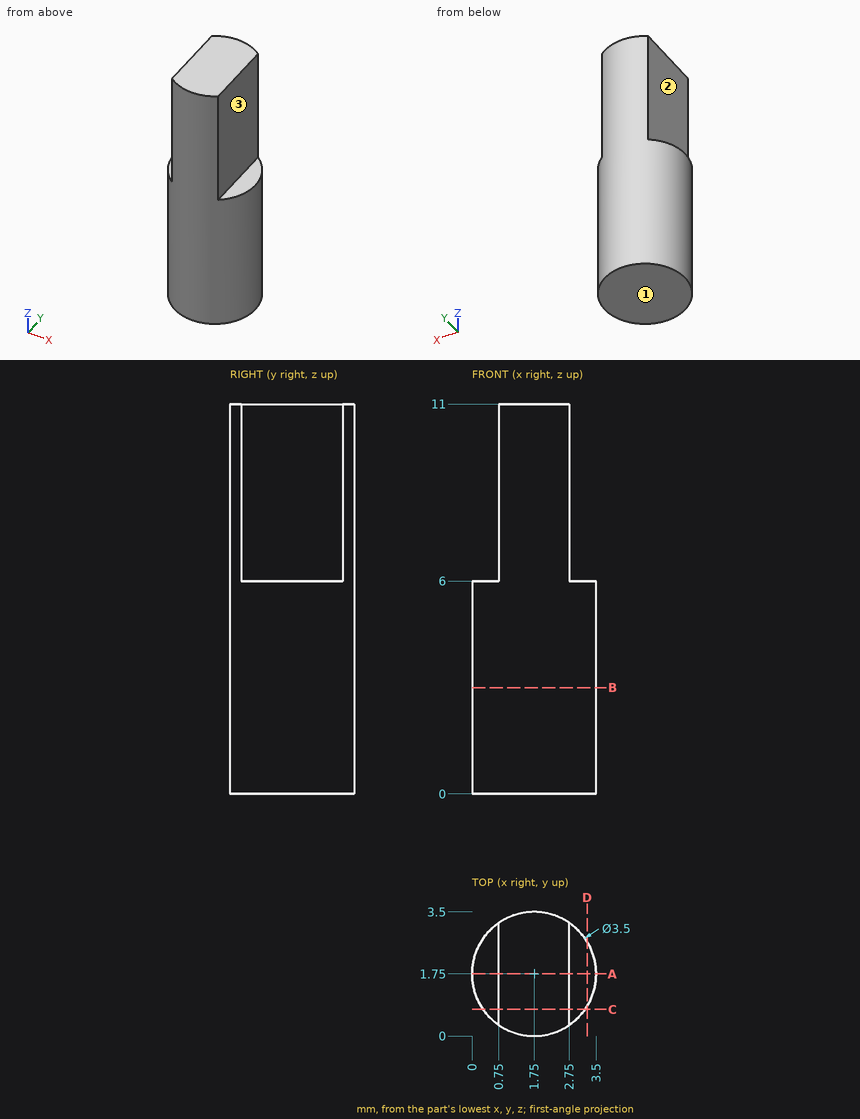
Input: dimensioned drawing with shaded views. Units: mm. Origin: part minimum x, y, z. A direction names the side the tool comes from. Give positions to 0.01 mm unless a question says otherwise; leave off trailing zeros. Loops run counter-clockwise (first coordinate to the right, second up) from the corner with the lowest first, then second, coordinate; pieces in that order, holes last. Notation, with made-up numbers: M 34,31 L 93,31 A19 cw 93,36 Z; hole C 2.25,0.5 d1. An arc over 180 degrees is marked long. Put each result on its own line as item: value. Start each with the question number.
1) Cut plane C-C (y = 0.75). Output: boundary loops of the cut face in (x, z), then the cut area to 3 significant figures.
2) Cut plane D-D (x = 3.25). Output: boundary loops of the cut face in (y, z), then the cut area to 3 significant figures.
3) Ray query, line 1 along X through (y, z) = (0.35, 10.25); line 2 along Z through (x, y) = (3.15, 1.2); line 3 along Y through (x, z) = (1.65, 6.5). Return the intervals inside material, ascending.
4) Contact query for a flat-ended pin moving along its axis: pin 1 (2 mm diameter, centred on y = 0.5, z = 9.5, fed in from +X). Output: stop coordinate, or through.
5) Access query for the marked faces 1, 2 and 3. Directions: +Z, -Z, +X, -X, +Y, -Y. A direction counts if a zero-diameter tool reaches every point of the face in a straight line with its end or side. Return the directions, or none.
6) Cut plane B-B (z = 3). Output: boundary loops of the cut face in (x, y), then the cut area to 3 significant figures.
7) Cut plane A-A (y = 1.75). Output: boundary loops of the cut face in (x, z), then the cut area to 3 significant figures.
Verdict:
1. outline: M 0.31,0 L 3.19,0 L 3.19,6 L 2.75,6 L 2.75,11 L 0.75,11 L 0.75,6 L 0.31,6 Z
1. area: 27.2 mm2
2. outline: M 0.85,0 L 2.65,0 L 2.65,6 L 0.85,6 Z
2. area: 10.8 mm2
3. line 1: 0.75 to 2.75
3. line 2: 0 to 6
3. line 3: 0 to 3.5
4. pin 1: x = 2.75
5. face 1: -Z, +X, -X, +Y, -Y
5. face 2: +Z, -X, +Y, -Y
5. face 3: +Z, +X, +Y, -Y
6. outline: C 1.75,1.75 d3.5
6. area: 9.62 mm2
7. outline: M 0,0 L 3.5,0 L 3.5,6 L 2.75,6 L 2.75,11 L 0.75,11 L 0.75,6 L 0,6 Z
7. area: 31.0 mm2
